Geometry check sheet. Reference: the model listing, model coordinates, mm. A direction names the side the tool comes from. Round coordinates to 2 decimals unless told otherwise and drop trailing zeros. Loops run counter-clockwise (first coordinate to the right, second up) from the corner with the lowest first, then second, coordinate; pieces in that order, holes last. Notation, with made-up numbers: (29.25, -21) -> (37.25, -21) arc R20 ccw to (37.25, 5) -> close; hole circle Ø11 at (72.5, -25). An arc over 180 degrees is marked (long way). Use a Markdown table: item, result. Add a question column.
Q1. Sectioned sample at A-A, the plane x = 42.25. Enter the section's corners in (y, z).
Q2. Set-up check for faces 1 (the face through (-55.78, 25.14, 63.23)), 2 (the face through (-5.959, 18.269, 5.332)), 3 (the face through (-17, 35, -1)): record each of +Z, -Z, +X, -X, +Y, -Y from which the full face is reachable in a straight line by a thin tool's end or side.
Q3. Sectioned sample at B-B, the plane y = 24. Give the number of separate pieces and of enclosed holes in the cut face, then the cut area to 3 significant figures.
Q4. Gauge pin test, flat end, axial feed: P1, Ø15, axis at x = 45, z = -56.5, coming from the +Y side. Record the tip position at first contact, or that the pin passes through.
Q5. Sectioned sample at D-D, the plane z = -7. Enter the section's corners in (x, y).
Q6. Material ranges on L1, parallel to X at y = 12.25, z = -56.19; L2, parallel to X at y = 29.75, z = -56.19; L3, parallel to Z at x = 42, y = 25, recorded low to high.
Q7. Sectioned sample at C-C, the plane x = 10.25. Enter the section's corners in (y, z).
Q8. Release check for a two-part mould opening along Z. For faces 4 (the face through (-39, 15, -46)), 5 (the face through (72.25, 17, 1)) record: released by +Z, released by -Z, zero draft, split by the parting line, or undercut.
```python
from build123d import *

# Parameters (mm, degrees)
SKETCH1_W           = 144.5
SKETCH1_H           = 172.38
BOSS_EXTRUDE1_DEPTH = 35
CUT_EXTRUDE1_REACH  = 119.787
SKETCH2_R           = 1.99
SKETCH2_R_2         = 10.5
CUT_EXTRUDE2_DEPTH  = 2
SKETCH4_R           = 15.25
CUT_EXTRUDE3_DEPTH  = 20


with BuildPart() as part:
    # Sketch1 → Boss-Extrude1 (new body)
    with BuildSketch(Plane(origin=(0, 0, 0), x_dir=(1, 0, 0), z_dir=(0, 1, 0))):
        Rectangle(SKETCH1_W, SKETCH1_H)
    extrude(amount=BOSS_EXTRUDE1_DEPTH)

    # Sketch2 → Cut-Extrude1 (cut, up to next)
    with BuildSketch(Plane.XZ, mode=Mode.PRIVATE) as cut_extrude1_sk1:
        with Locations(Location((10.25, -56.19, 0), (0, 0, 270))):
            Circle(SKETCH2_R)
    cut_extrude1_tool1 = extrude(cut_extrude1_sk1.sketch, amount=-CUT_EXTRUDE1_REACH, mode=Mode.PRIVATE) & part.part
    # Sketch2 → Cut-Extrude1 (cut, up to next)
    with BuildSketch(Plane.XZ, mode=Mode.PRIVATE) as cut_extrude1_sk2:
        with Locations(Location((-42.25, -56.19, 0), (0, 0, 270))):
            Circle(SKETCH2_R_2)
    cut_extrude1_tool2 = extrude(cut_extrude1_sk2.sketch, amount=-CUT_EXTRUDE1_REACH, mode=Mode.PRIVATE) & part.part
    # Sketch2 → Cut-Extrude1 (cut, up to next)
    with BuildSketch(Plane.XZ, mode=Mode.PRIVATE) as cut_extrude1_sk3:
        with Locations(Location((42.25, -56.19, 0), (0, 0, 270))):
            Circle(SKETCH2_R_2)
    cut_extrude1_tool3 = extrude(cut_extrude1_sk3.sketch, amount=-CUT_EXTRUDE1_REACH, mode=Mode.PRIVATE) & part.part
    # Sketch2 → Cut-Extrude1 (cut, up to next)
    with BuildSketch(Plane.XZ, mode=Mode.PRIVATE) as cut_extrude1_sk4:
        with Locations(Location((-42.25, 56.19, 0), (0, 0, 270))):
            Circle(SKETCH2_R_2)
    cut_extrude1_tool4 = extrude(cut_extrude1_sk4.sketch, amount=-CUT_EXTRUDE1_REACH, mode=Mode.PRIVATE) & part.part
    # Sketch2 → Cut-Extrude1 (cut, up to next)
    with BuildSketch(Plane.XZ, mode=Mode.PRIVATE) as cut_extrude1_sk5:
        with Locations(Location((-10.25, 56.19, 0), (0, 0, 270))):
            Circle(SKETCH2_R)
    cut_extrude1_tool5 = extrude(cut_extrude1_sk5.sketch, amount=-CUT_EXTRUDE1_REACH, mode=Mode.PRIVATE) & part.part
    # Sketch2 → Cut-Extrude1 (cut, up to next)
    with BuildSketch(Plane.XZ, mode=Mode.PRIVATE) as cut_extrude1_sk6:
        with Locations(Location((42.25, 56.19, 0), (0, 0, 270))):
            Circle(SKETCH2_R_2)
    cut_extrude1_tool6 = extrude(cut_extrude1_sk6.sketch, amount=-CUT_EXTRUDE1_REACH, mode=Mode.PRIVATE) & part.part
    # Sketch2 → Cut-Extrude1 (cut, up to next)
    with BuildSketch(Plane.XZ, mode=Mode.PRIVATE) as cut_extrude1_sk7:
        Polygon((57.25, -20.94), (67.25, -20.94), (67.25, -17.44), (65.25, -17.44), (65.25, -17.94), (59.25, -17.94), (59.25, -17.44), (57.25, -17.44), align=None)
    cut_extrude1_tool7 = extrude(cut_extrude1_sk7.sketch, amount=-CUT_EXTRUDE1_REACH, mode=Mode.PRIVATE) & part.part
    # Sketch2 → Cut-Extrude1 (cut, up to next)
    with BuildSketch(Plane.XZ, mode=Mode.PRIVATE) as cut_extrude1_sk8:
        with BuildLine():
            Line((-1.333860018, -0.707106781), (-10.455537495, -9.828784258))
            ThreePointArc((-10.455537495, -9.828784258), (-10.455537495, -13.647160877), (-6.637160877, -13.647160877))
            Line((-6.637160877, -13.647160877), (7.01, 0))
            Line((7.01, 0), (-6.637160877, 13.647160877))
            ThreePointArc((-6.637160877, 13.647160877), (-10.455537495, 13.647160877), (-10.455537495, 9.828784258))
            Line((-10.455537495, 9.828784258), (-1.333860018, 0.707106781))
            ThreePointArc((-1.333860018, 0.707106781), (0.373246763, 0), (-1.333860018, -0.707106781))
        make_face()
    cut_extrude1_tool8 = extrude(cut_extrude1_sk8.sketch, amount=-CUT_EXTRUDE1_REACH, mode=Mode.PRIVATE) & part.part
    add(cut_extrude1_tool1.solids().sort_by_distance((10.25, 0, -56.19))[0], mode=Mode.SUBTRACT)
    add(cut_extrude1_tool2.solids().sort_by_distance((-42.25, 0, -56.19))[0], mode=Mode.SUBTRACT)
    add(cut_extrude1_tool3.solids().sort_by_distance((42.25, 0, -56.19))[0], mode=Mode.SUBTRACT)
    add(cut_extrude1_tool4.solids().sort_by_distance((-42.25, 0, 56.19))[0], mode=Mode.SUBTRACT)
    add(cut_extrude1_tool5.solids().sort_by_distance((-10.25, 0, 56.19))[0], mode=Mode.SUBTRACT)
    add(cut_extrude1_tool6.solids().sort_by_distance((42.25, 0, 56.19))[0], mode=Mode.SUBTRACT)
    add(cut_extrude1_tool7.solids().sort_by_distance((62.25, 0, -19.330625))[0], mode=Mode.SUBTRACT)
    add(cut_extrude1_tool8.solids().sort_by_distance((-0.05515, 0, -6.582011))[0], mode=Mode.SUBTRACT)

    # Sketch3 → Cut-Extrude2 (cut)
    with BuildSketch(Plane.XZ):
        Polygon((-72.25, 17.44), (-72.25, -17.94), (57.25, -17.94), (57.25, -20.94), (72.25, -20.94), (72.25, -19.644727293), (72.25, 17.44), align=None)
    extrude(amount=-CUT_EXTRUDE2_DEPTH, mode=Mode.SUBTRACT)

    # Sketch4 → Cut-Extrude3 (cut)
    with BuildSketch(Plane(origin=(0, 35, 0), x_dir=(1, 0, 0), z_dir=(0, 1, 0))):
        with Locations(Location((-42.25, 56.19, 0), (0, 0, 270))):
            Circle(SKETCH4_R)
        with Locations(Location((42.25, 56.19, 0), (0, 0, 270))):
            Circle(SKETCH4_R)
        with Locations(Location((42.25, -56.19, 0), (0, 0, 270))):
            Circle(SKETCH4_R)
        with Locations(Location((-42.25, -56.19, 0), (0, 0, 270))):
            Circle(SKETCH4_R)
    extrude(amount=-CUT_EXTRUDE3_DEPTH, mode=Mode.SUBTRACT)


solid = part.part
```
Values:
| question | item | result |
|---|---|---|
| 1 | outline | (0, -86.19) -> (35, -86.19) -> (35, -71.44) -> (15, -71.44) -> (15, -66.69) -> (0, -66.69) -> close; (0, -45.69) -> (15, -45.69) -> (15, -40.94) -> (35, -40.94) -> (35, 40.94) -> (15, 40.94) -> (15, 45.69) -> (0, 45.69) -> (0, 17.44) -> (2, 17.44) -> (2, -17.94) -> (0, -17.94) -> close; (0, 66.69) -> (15, 66.69) -> (15, 71.44) -> (35, 71.44) -> (35, 86.19) -> (0, 86.19) -> close |
| 2 | face 1 | +Y |
| 2 | face 2 | +Y, -Y |
| 2 | face 3 | +Z, -Z, +X, -X, +Y |
| 3 | separate pieces | 1 |
| 3 | enclosed holes | 8 |
| 3 | area | 21,700 mm^2 |
| 4 | P1 | through |
| 5 | outline | (-72.25, 2) -> (-7.63, 2) -> (-7.63, 35) -> (-72.25, 35) -> close; (0.01, 2) -> (72.25, 2) -> (72.25, 35) -> (0.01, 35) -> close |
| 6 | L1 | -72.25 to -52.75, -31.75 to 8.26, 12.24 to 31.75, 52.75 to 72.25 |
| 6 | L2 | -72.25 to -57.5, -27 to 8.26, 12.24 to 27, 57.5 to 72.25 |
| 6 | L3 | -86.19 to -71.44, -40.94 to 40.94, 71.44 to 86.19 |
| 7 | outline | (0, -86.19) -> (35, -86.19) -> (35, -58.18) -> (0, -58.18) -> close; (0, -54.2) -> (35, -54.2) -> (35, 86.19) -> (0, 86.19) -> (0, 17.44) -> (2, 17.44) -> (2, -17.94) -> (0, -17.94) -> close |
| 8 | face 4 | undercut |
| 8 | face 5 | zero draft |
